For this review, use the dimensioned drawing (mm, ordinates from the lowest corner) and the shaded views. Round coordinates to 2 decimals unless told otherwise and drop trailing zeros. Loops run counter-clockwise (first coordinate to the right, second up) from the corner with the lowest first, then second, coordinate; pieces in that order, holes last. Notation, with made-up numbers: M 62,72 L 80,72 A32 ccw 80,105 Z; hole C 81,58 d9. An arc over 180 degrees is marked long. Answer as a JSON object with one key per item and string values. Group by question number.
Item 1: Consider section D-D (x = 146). Give the boundary of the cut face in (y, z).
Item 2: Consider section B-B (z = 88). Give the boundary of the cut face in (x, y).
Item 3: Insertion check: P1, Ø2, axis at y = 132.5, z = 13, coming from the +X side; P2, Ø14, axis at x = 139, y = 7.5, coming from the -Z side; P3, Ø4, axis at x = 71, z = 29, coming from the +Y side. Each pin has a flat end and moves straight along its axis. Give the tip position at first contact, or say it passes through.
Item 4: Consider section C-C (y = 88). Give the boundary of the cut face in (x, z), and give its area (3 significant figures).
Item 5: To check wall thickness, follow line 1 (Y direction, x = 85, z = 120); line 2 (Z direction, x = 16, y = 8); line 3 (X direction, y = 174.5, z = 89). State the ranges of each line that lie inside material, in increasing order.
Item 6: Consider section A-A (x = 112). Give the boundary of the cut face in (y, z), and give its area (3 significant figures).
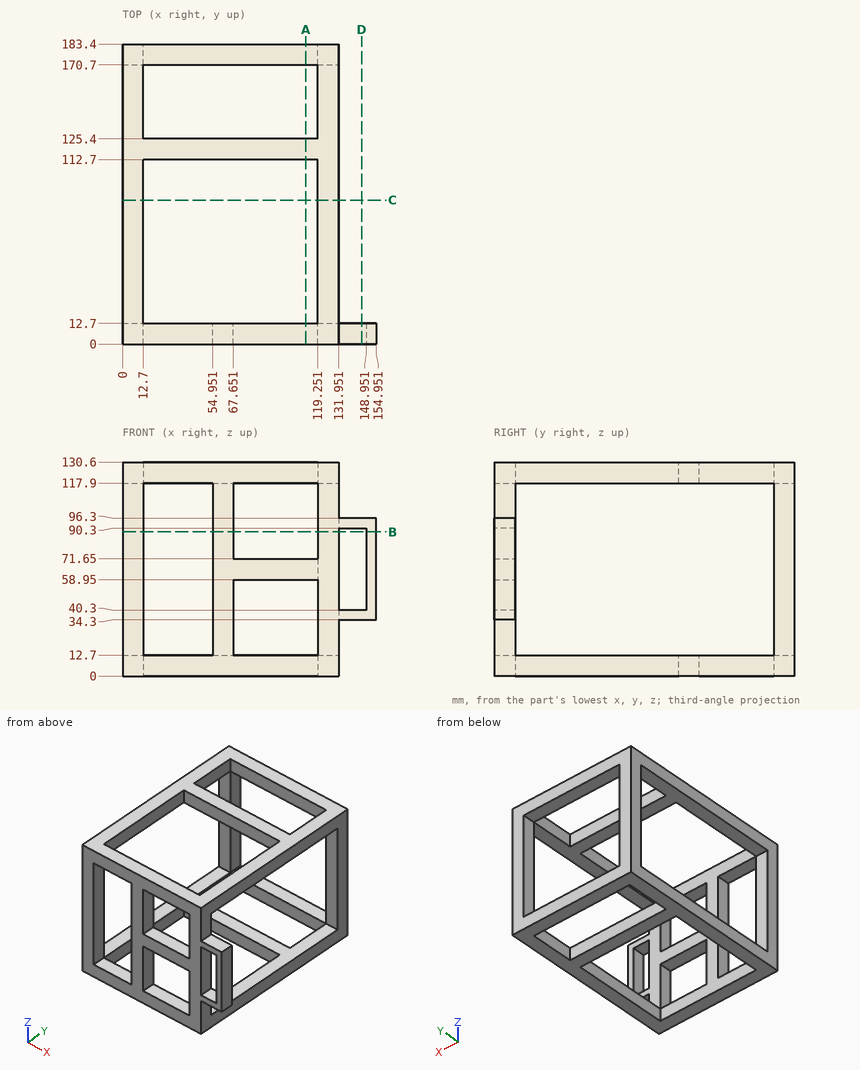
Geometry results:
{
 "1": {"outline": "M 0,34.3 L 12.7,34.3 L 12.7,40.3 L 0,40.3 Z; M 0,90.3 L 12.7,90.3 L 12.7,96.3 L 0,96.3 Z"},
 "2": {"outline": "M 0,0 L 12.7,0 L 12.7,12.7 L 0,12.7 Z; M 0,170.7 L 12.7,170.7 L 12.7,183.4 L 0,183.4 Z; M 54.95,0 L 67.65,0 L 67.65,12.7 L 54.95,12.7 Z; M 119.25,0 L 131.95,0 L 131.95,12.7 L 119.25,12.7 Z; M 119.25,170.7 L 131.95,170.7 L 131.95,183.4 L 119.25,183.4 Z; M 148.95,0 L 154.95,0 L 154.95,12.7 L 148.95,12.7 Z"},
 "3": {"P1": "stops at x = 131.95", "P2": "stops at z = 34.3", "P3": "passes through"},
 "4": {"outline": "M 0,0 L 12.7,0 L 12.7,12.7 L 0,12.7 Z; M 0,117.9 L 12.7,117.9 L 12.7,130.6 L 0,130.6 Z; M 119.25,0 L 131.95,0 L 131.95,12.7 L 119.25,12.7 Z; M 119.25,117.9 L 131.95,117.9 L 131.95,130.6 L 119.25,130.6 Z", "area": "645 mm^2"},
 "5": {"line 1": "y = 0 to 12.7, 112.7 to 125.4, 170.7 to 183.4", "line 2": "z = 0 to 12.7, 117.9 to 130.6", "line 3": "x = 0 to 12.7, 119.25 to 131.95"},
 "6": {"outline": "M 0,0 L 12.7,0 L 12.7,12.7 L 0,12.7 Z; M 0,58.95 L 12.7,58.95 L 12.7,71.65 L 0,71.65 Z; M 0,117.9 L 12.7,117.9 L 12.7,130.6 L 0,130.6 Z; M 112.7,0 L 125.4,0 L 125.4,12.7 L 112.7,12.7 Z; M 112.7,117.9 L 125.4,117.9 L 125.4,130.6 L 112.7,130.6 Z; M 170.7,0 L 183.4,0 L 183.4,12.7 L 170.7,12.7 Z; M 170.7,117.9 L 183.4,117.9 L 183.4,130.6 L 170.7,130.6 Z", "area": "1,130 mm^2"}
}
